The listing builds one solid part. Answer for the finished solid, in the listing's coordinates (mm). Round coordinates to 2 decimals unless told otherwise and drop trailing zeros. Write each loop counter-clockwise with the first axis right and the second up, starting at its lowest first coordinate (ties: lowest second). Pieces come first, ordered by that corner, then holes. Notation, with made-up numbers: M 17.25,3 L 67.25,3 A14 ccw 67.25,27 Z; hole C 20,19.5 d9. An arc over 180 degrees is marked long. Answer as CSV lines item,"result". Start each with the question number.
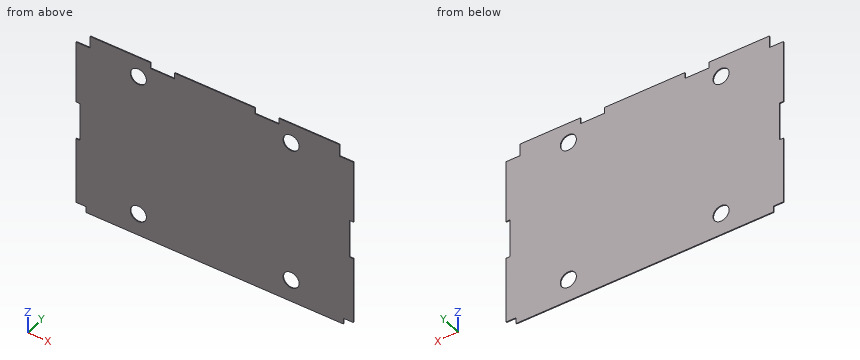
from build123d import *

# Parameters (mm, degrees)
SKETCH1_R           = 25.4
BOSS_EXTRUDE1_DEPTH = 2.65684


with BuildPart() as part:
    # Sketch1 → Boss-Extrude1 (new body)
    with BuildSketch(Plane(origin=(0, 0, 0), x_dir=(1, 0, 0), z_dir=(0, 1, 0))):
        Polygon((-438.15, 273.05), (-406.4, 273.05), (-406.4, 292.1), (406.4, 292.1), (406.4, 273.05), (438.15, 273.05), (438.15, 63.5), (425.45, 63.5), (425.45, -57.15), (438.15, -57.15), (438.15, -254), (393.7, -254), (393.7, -292.1), (203.2, -292.1), (203.2, -273.05), (127, -273.05), (127, -292.1), (-127, -292.1), (-127, -273.05), (-203.2, -273.05), (-203.2, -292.1), (-393.7, -292.1), (-393.7, -254), (-438.15, -254), (-438.15, -57.15), (-425.45, -57.15), (-425.45, 63.5), (-438.15, 63.5), align=None)
        with Locations((241.3, 222.25)):
            Circle(SKETCH1_R, mode=Mode.SUBTRACT)
        with Locations((241.3, -228.6)):
            Circle(SKETCH1_R, mode=Mode.SUBTRACT)
        with Locations((-241.3, 222.25)):
            Circle(SKETCH1_R, mode=Mode.SUBTRACT)
        with Locations((-241.3, -228.6)):
            Circle(SKETCH1_R, mode=Mode.SUBTRACT)
    extrude(amount=BOSS_EXTRUDE1_DEPTH)


solid = part.part
Q1. Find section D-D (z = -40.5). Determine the outline of the cut face in (x, y).
Q2. Straight lines are drawn through the part: L1, parallel to Z at x = 241.3, y = 1.5; L2, parallel to X at y = 2, z = -222.25; L3, parallel to X at y = 2.5, z = -243.5. For each, find the intervals that lie inside material, in ascending order.
Q3. Find section A-A (y = 0.5). Count the separate pieces of the cut face and the enclosed holes in it, plus the area to 3 significant figures.
Q4. Each of these flat-tipped pins is pushed along its axis until it touches: P1, Ø0.8, axis at x = 429, y = 1, coming from the -Z side; P2, Ø1.3, axis at y = 1.5, z = -286.5, coming from the +X side; P3, Ø1.5, axis at x = -101.5, z = -174.5, coming from the -Y side; P4, Ø0.8, axis at x = 405.5, y = 1.5, coming from the +Z side. Where does it stop, or does it pass through?
Q5. Find section C-C (x = -241.3). Determine the outline of the cut face in (y, z).
Q6. Find section B-B (z = 228.6). Determine the outline of the cut face in (x, y), plus the area to 3 significant figures.
Reported:
1,outline,"M -425.45,0 L 425.45,0 L 425.45,2.66 L -425.45,2.66 Z"
2,L1,"z = -292.1 to -247.65, -196.85 to 203.2, 254 to 292.1"
2,L2,"x = -438.15 to -266.7, -215.9 to 215.9, 266.7 to 438.15"
2,L3,"x = -438.15 to -255.21, -227.39 to 227.39, 255.21 to 438.15"
3,separate pieces,"1"
3,enclosed holes,"4"
3,area,"493,000 mm2"
4,P1,"stops at z = -273.05"
4,P2,"stops at x = 406.4"
4,P3,"stops at y = 0"
4,P4,"stops at z = 254"
5,outline,"M 0,-292.1 L 2.66,-292.1 L 2.66,-247.65 L 0,-247.65 Z; M 0,-196.85 L 2.66,-196.85 L 2.66,203.2 L 0,203.2 Z; M 0,254 L 2.66,254 L 2.66,292.1 L 0,292.1 Z"
6,outline,"M -438.15,0 L -266.7,0 L -266.7,2.66 L -438.15,2.66 Z; M -215.9,0 L 215.9,0 L 215.9,2.66 L -215.9,2.66 Z; M 266.7,0 L 438.15,0 L 438.15,2.66 L 266.7,2.66 Z"
6,area,"2,060 mm2"
